Design review of the part built by this model. Coordinates are the model's own, in mm. Face numbers are marked on the shaded views. A direction names the side the tool comes from. Coordinates: 2 decimals unless noted, no trailing zeros. Write each loop counter-clockwise with the first axis right and the second up, starting at its lowest first coordinate (ties: lowest second). Pieces come first, ordered by that corner, then holes. Notation, with made-up numbers: (-13.5, 81.5) - (-1.5, 81.5) arc R13 ccw to (-1.5, 92.5) - close; hole circle Ø7 at (-35.75, -26.5). An arc over 180 degrees is marked (long way). Answer as a JSON object with one key per item and string values.
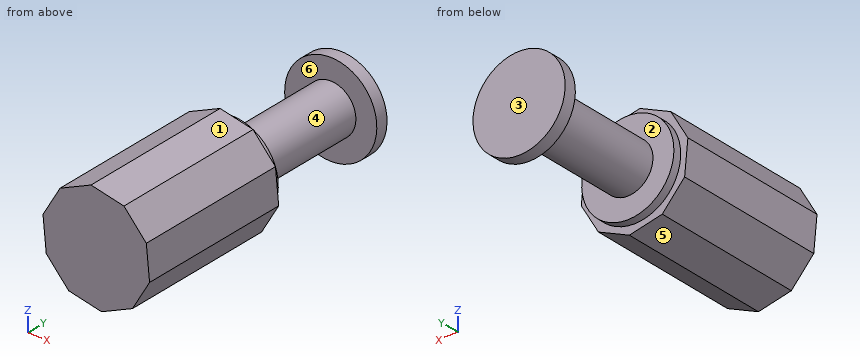
```python
from build123d import *

# Parameters (mm, degrees)
EXTRUDE_2_DEPTH = 190


with BuildPart() as part:
    # Эскиз2 → Повернуть1 (revolve)
    with BuildSketch(Plane(origin=(0, 0, 0), x_dir=(0, 0, -1), z_dir=(1, 0, 0))):
        Polygon((0, 0), (55, 0), (55, 10), (30, 10), (30, 155), (55, 155), (55, 170), (0, 170), align=None)
    revolve(axis=Axis((0, -61.701185429, 0), (0, 1, 0)))

    # Эскиз3 → Бобышка-Вытянуть2 (add)
    with BuildSketch(Plane.XZ):
        Polygon((43.193084505, -48.718094896), (63.579717104, -14.025508632), (59.681058764, 26.024345221), (32.986264461, 56.133783734), (-6.308161704, 64.802024777), (-43.193084505, 48.718094896), (-63.579717104, 14.025508632), (-59.681058764, -26.024345221), (-32.986264461, -56.133783734), (6.308161704, -64.802024777), align=None)
    extrude(amount=EXTRUDE_2_DEPTH)


solid = part.part
```
(1) Take a section at C-C, the plane z = 0. Write out the cut boundary in (x, y).
Solved:
{"outline": "(-62.21, -190) - (62.21, -190) - (62.21, 0) - (55, 0) - (55, 10) - (30, 10) - (30, 155) - (55, 155) - (55, 170) - (-55, 170) - (-55, 155) - (-30, 155) - (-30, 10) - (-55, 10) - (-55, 0) - (-62.21, 0) - close"}
(2) Tool access review of the marked faces 1 and 2: name each direction out of +Z, -Z, +X, -X, +Y, -Y from which nothing blocks a thin tool from reaching the whole face with its end or side.
Solved:
{"face 1": "+Z, +X, +Y, -Y", "face 2": "none"}
(3) To check wall thickness, follow line 1 (Y direction, x = 39, z = -24.5); line 2 (Y direction, x = -33.5, z = -51); line 3 (Z direction, x = 27.5, y = -97.5). State the ranges of each line that lie inside material, in increasing order. Write a range as from..to.
Solved:
{"line 1": "y = -190..10, 155..170", "line 2": "y = -190..0", "line 3": "z = -55.56..57.34"}
(4) Take a section at D-D, the plane y = 19.5. Write out the cut boundary in (x, z).
Solved:
{"outline": "circle Ø60 at (0, 0)"}
(5) Take a section at A-A, the plane y = -37. Write out the cut boundary in (x, z).
Solved:
{"outline": "(-63.58, 14.03) - (-59.68, -26.02) - (-32.99, -56.13) - (6.31, -64.8) - (43.19, -48.72) - (63.58, -14.03) - (59.68, 26.02) - (32.99, 56.13) - (-6.31, 64.8) - (-43.19, 48.72) - close"}
(6) Take a section at B-B, the plane x = 22. Write out the cut boundary in (y, z), and give its area (3 significant figures).
Solved:
{"outline": "(-190, -57.96) - (0, -57.96) - (0, -50.41) - (10, -50.41) - (10, -20.4) - (155, -20.4) - (155, -50.41) - (170, -50.41) - (170, 50.41) - (155, 50.41) - (155, 20.4) - (10, 20.4) - (10, 50.41) - (0, 50.41) - (0, 58.56) - (-190, 58.56) - close", "area": "30,600 mm^2"}
(7) For pin 1 (3 mm diameter, centred on y = -45, z = 35.5, fed in from -X); pin 2 (12 mm diameter, centred on y = 112.5, z = 33, fed in from +X); pin 3 (1 mm diameter, centred on y = -10, z = -6, fed in from +X), all flat-tipped, find the tip position at first contact; note any pin that passes through.
Solved:
{"pin 1": "stops at x = -51.84", "pin 2": "stops at x = 13.08", "pin 3": "stops at x = 62.85"}
(8) The part is to be moulded in two halves that separate along Y. For the marked faces 3, 4, 5 and 6, say which applies: pulls with the +Y half, pulls with the -Y half, needs draft (parallel to the pull), parting line crosses it, or undercut.
Solved:
{"face 3": "pulls with the +Y half", "face 4": "undercut", "face 5": "needs draft", "face 6": "undercut"}
